from build123d import *

# Parameters (mm, degrees)
F2_R = 5.08


with BuildPart() as f1:
    # F0 (on Front) → F1 (revolve)
    with BuildSketch(Plane.XZ):
        with BuildLine():
            Line((37.5, 6.25), (0, 6.25))
            Line((0, 6.25), (-37.5, 6.25))
            ThreePointArc((-37.5, 6.25), (-42.92127, 7.847034), (-46.610949, 12.128033))
            Line((-46.610949, 12.128033), (-80.26316, 12.128033))
            Line((-80.26316, 12.128033), (-80.26316, 0))
            Line((-80.26316, 0), (80.26316, 0))
            Line((80.26316, 0), (80.26316, 12.128033))
            Line((80.26316, 12.128033), (46.610949, 12.128033))
            ThreePointArc((46.610949, 12.128033), (42.92127, 7.847034), (37.5, 6.25))
        make_face()
    revolve(axis=Axis((0, 0, 0), (1, 0, 0)))

    # F2
    f2_edges = [f1.edges().sort_by_distance(p)[0] for p in [
        (-37.5, 0, -6.25),
        (-46.610949, 0, -12.128033),
        (-42.92127, 0, 7.847034),
        (46.610949, 0, -12.128033),
        (37.5, 0, -6.25),
        (-80.26316, 0, -12.128033),
        (80.26316, 0, -12.128033),
    ]]
    fillet(f2_edges, radius=F2_R)


solid = f1.part
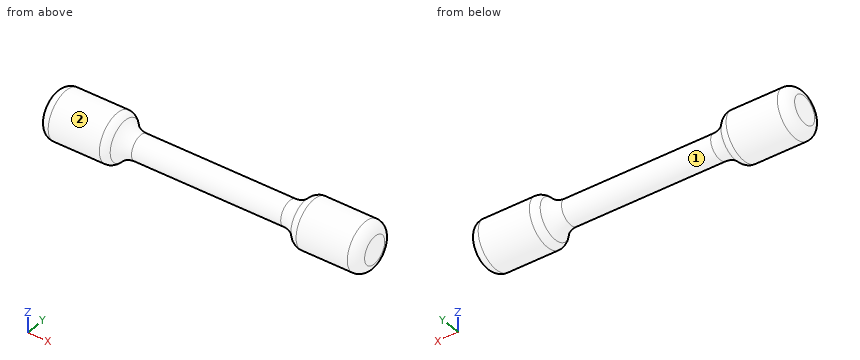
Can you work these out from the model? Positions are in its coordinate system, mm. Face numbers are marked on the shaded views. A direction names the side the tool comes from. Round coordinates to 2 decimals unless told otherwise and drop trailing zeros. Loops run counter-clockwise (first coordinate to the right, second up) from the corner with the lowest first, then second, coordinate; pieces in that order, holes last. Notation, with made-up numbers: (-29.75, -15.75) - (28.25, -15.75) arc R12 ccw to (28.25, 1.25) - close; hole circle Ø1 at (-10, 89). An arc over 180 degrees is marked (long way). Use CSV: the item, a comma, the result in double quotes. Start each with the question number.
1) Please list where these lines run through material, in increasing order: probe 1 along Z at (x, y) = (-60.5, -0.75); probe 2 along X at (y, z) = (0.25, -7.75); probe 3 along X at (y, z) = (8.5, -2.25). Write a range as [from, to].
2) For pin 1 Ø12 at (x, y) = (19.5, 0.5) entering from -Z; pin 2 Ø4 at (x, z) = (45.5, -3) entering from +Y; pin 3 Ø10 at (x, z) = (-57, -9.5) entering from -Y, each with a flat end and sliding along its axis, tell me the tip position at first contact or that it passes through.
3) If we section it at A-A on x = -56: Write out the boundary of the cut face in (y, z).
4) If we section it at B-B on x = 1: Write out the boundary of the cut face in (y, z).
5) For the marked faces 1 and 2, which set-ups out of +Z, -Z, +X, -X, +Y, -Y let a thin tool reach every point of the face, with its end or its side?
Geometry results:
1,probe 1,"z = [-12.1, 12.1]"
1,probe 2,"x = [-80.21, -42.77], [42.77, 80.21]"
1,probe 3,"x = [-79.95, -44.16], [44.16, 79.95]"
2,pin 1,"stops at z = -6.25"
2,pin 2,"stops at y = 11.46"
2,pin 3,"stops at y = -11.26"
3,outline,"circle Ø24.26 at (0, 0)"
4,outline,"circle Ø12.5 at (0, 0)"
5,face 1,"none"
5,face 2,"+X, -X"
